Geometry check sheet. Reference: the model listing, model coordinates, mm. A direction names the side the tool comes from. Round coordinates to 2 decimals unless told otherwise and drop trailing zeros. Loops run counter-clockwise (first coordinate to the right, second up) from the corner with the lowest first, then second, coordinate; pieces in that order, holes last.
```python
from build123d import *

# Parameters (mm, degrees)
SKETCH1_W               = 68.58
SKETCH1_H               = 57.15
BOSS_EXTRUDE1_DEPTH     = 31.75
SKETCH2_W               = 26.162
SKETCH2_H               = 26.162
SKETCH2_W_2             = 26.67
SKETCH2_H_2             = 27.94
CUT_EXTRUDE1_DEPTH      = 95.749149864
SKETCH5_R               = 3.556
SKETCH5_R_2             = 3.729278609
CUT_EXTRUDE2_DEPTH      = 95.749149864
CUT_EXTRUDE3_START      = -16.51
CUT_EXTRUDE3_DEPTH      = 6.35
SKETCH7_R               = 5.334
CUT_EXTRUDE4_DEPTH      = 5.842
CUT_EXTRUDE5_DEPTH      = 7.62
SKETCH10_W              = 36.322
SKETCH10_H              = 6.35
CUT_EXTRUDE6_DEPTH      = 95.749149864
CUT_EXTRUDE7_DEPTH      = 87.293112332
CUT_EXTRUDE7_DEPTH_BACK = 87.293112332
SKETCH12_R              = 3.556
SKETCH13_R              = 5.334
CUT_EXTRUDE8_DEPTH      = 6.35
CUT_EXTRUDE9_DEPTH      = 7.62
CHAMFER1_SIZE           = 0.762
CHAMFER3_SIZE           = 3.81
CHAMFER5_SIZE           = 1.27
CHAMFER6_SIZE           = 2.54
CHAMFER9_SIZE           = 3.81
CHAMFER10_SIZE          = 6.35


# Some blends are built 0.0001 mm under size
with BuildPart() as part:
    # Sketch1 → Boss-Extrude1 (new body)
    with BuildSketch(Plane.XY):
        with Locations((34.29, 28.575)):
            Rectangle(SKETCH1_W, SKETCH1_H)
    extrude(amount=BOSS_EXTRUDE1_DEPTH)

    # Sketch2 → Cut-Extrude1 (cut, through all)
    with BuildSketch(Plane.XY.offset(31.75)):
        with Locations((19.431, 28.575)):
            Rectangle(SKETCH2_W, SKETCH2_H)
        with Locations((49.022, 28.575)):
            Rectangle(SKETCH2_W_2, SKETCH2_H_2)
    extrude(amount=-CUT_EXTRUDE1_DEPTH, mode=Mode.SUBTRACT)

    # Sketch5 → Cut-Extrude2 (cut, through all)
    with BuildSketch(Plane(origin=(68.58, 0, 0), x_dir=(0, 0, -1), z_dir=(1, 0, 0))):
        with Locations((-12.7, 47.625)):
            Circle(SKETCH5_R)
        with Locations((-12.7, 9.525)):
            Circle(SKETCH5_R_2)
    extrude(amount=-CUT_EXTRUDE2_DEPTH, mode=Mode.SUBTRACT)

    # Sketch6 → Cut-Extrude3 (cut)
    with BuildSketch(Plane(origin=(68.58, 0, 0), x_dir=(0, 0, -1), z_dir=(1, 0, 0)).offset(CUT_EXTRUDE3_START)):
        with BuildLine():
            Line((-21.59, 47.625), (-21.59, 12.21272508))
            ThreePointArc((-21.59, 12.21272508), (-15.38772508, 0.635), (-3.81, 6.83727492))
            Line((-3.81, 6.83727492), (-3.81, 47.625))
            ThreePointArc((-3.81, 47.625), (-12.7, 56.515), (-21.59, 47.625))
        make_face()
    extrude(amount=-CUT_EXTRUDE3_DEPTH, mode=Mode.SUBTRACT)

    # Sketch7 → Cut-Extrude4 (cut)
    with BuildSketch(Plane(origin=(68.58, 0, 0), x_dir=(0, 0, -1), z_dir=(1, 0, 0))):
        with Locations((-12.7, 47.625)):
            Circle(SKETCH7_R)
        with Locations((-12.7, 9.525)):
            Circle(SKETCH7_R)
    extrude(amount=-CUT_EXTRUDE4_DEPTH, mode=Mode.SUBTRACT)

    # Sketch9 → Cut-Extrude5 (cut)
    with BuildSketch(Plane.ZY):
        Polygon((16.072880273, 53.467), (9.327119727, 53.467), (5.954239455, 47.625), (9.327119727, 41.783), (16.072880273, 41.783), (19.445760545, 47.625), align=None)
        Polygon((16.072880273, 15.367), (9.327119727, 15.367), (5.954239455, 9.525), (9.327119727, 3.683), (16.072880273, 3.683), (19.445760545, 9.525), align=None)
    extrude(amount=-CUT_EXTRUDE5_DEPTH, mode=Mode.SUBTRACT)

    # Sketch10 → Cut-Extrude6 (cut, through all)
    with BuildSketch(Plane(origin=(0, 57.15, 0), x_dir=(1, 0, 0), z_dir=(0, 1, 0))):
        with Locations((50.419, -28.575)):
            Rectangle(SKETCH10_W, SKETCH10_H)
    extrude(amount=-CUT_EXTRUDE6_DEPTH, mode=Mode.SUBTRACT)

    # Sketch12 → Cut-Extrude7 (cut, two sides: drawn at the far end of the back side and taken through both)
    with BuildSketch(Plane(origin=(0, 15.494, 0), x_dir=(1, 0, 0), z_dir=(0, 1, 0)).offset(-CUT_EXTRUDE7_DEPTH_BACK)):
        with Locations(Location((19.431, -22.86, 0), (0, 0, 180))):
            Circle(SKETCH12_R)
    extrude(amount=CUT_EXTRUDE7_DEPTH + CUT_EXTRUDE7_DEPTH_BACK, mode=Mode.SUBTRACT)

    # Sketch13 → Cut-Extrude8 (cut)
    with BuildSketch(Plane(origin=(0, 57.15, 0), x_dir=(1, 0, 0), z_dir=(0, 1, 0))):
        with Locations(Location((19.431, -22.86, 0), (0, 0, 270))):
            Circle(SKETCH13_R)
    extrude(amount=-CUT_EXTRUDE8_DEPTH, mode=Mode.SUBTRACT)

    # Sketch14 → Cut-Extrude9 (cut)
    with BuildSketch(Plane.XZ):
        Polygon((22.803880273, 28.702), (16.058119727, 28.702), (12.685239455, 22.86), (16.058119727, 17.018), (22.803880273, 17.018), (26.176760545, 22.86), align=None)
    extrude(amount=-CUT_EXTRUDE9_DEPTH, mode=Mode.SUBTRACT)

    # Chamfer1
    chamfer1_edges = [part.edges().sort_by_distance(p)[0] for p in [
        (0, 50.546, 17.759320409),
        (0, 53.467, 12.7),
        (0, 50.546, 7.640679591),
        (0, 44.704, 7.640679591),
        (0, 41.783, 12.7),
        (0, 44.704, 17.759320409),
        (0, 12.446, 17.759320409),
        (0, 15.367, 12.7),
        (0, 12.446, 7.640679591),
        (0, 6.604, 7.640679591),
        (0, 3.683, 12.7),
        (0, 6.604, 17.759320409),
        (22.987, 41.656, 22.86),
        (22.987, 15.494, 22.86),
        (19.431, 57.15, 17.526),
        (24.490320409, 0, 25.781),
        (19.431, 0, 28.702),
        (14.371679591, 0, 25.781),
        (14.371679591, 0, 19.939),
        (19.431, 0, 17.018),
        (24.490320409, 0, 19.939),
        (45.72, 47.625, 16.256),
        (45.72, 9.525, 16.429278609),
        (52.07, 9.525, 16.429278609),
        (52.07, 47.625, 16.256),
        (68.58, 47.625, 18.034),
        (68.58, 9.525, 18.034),
    ]]
    chamfer(chamfer1_edges, length=CHAMFER1_SIZE)

    # Chamfer3
    chamfer3_edges = [part.edges().sort_by_distance(p)[0] for p in [
        (49.022, 42.545, 25.4),
        (49.022, 14.605, 25.4),
        (49.022, 42.545, 0),
        (49.022, 14.605, 0),
    ]]
    chamfer(chamfer3_edges, length=CHAMFER3_SIZE - 0.0001)  # a hair under: the kernel refuses the full size

    # Chamfer5
    chamfer5_edges = [part.edges().sort_by_distance(p)[0] for p in [
        (19.304, 41.656, 31.75),
        (32.258, 49.403, 31.75),
        (32.258, 7.747, 31.75),
        (35.687, 28.575, 25.4),
        (62.357, 28.575, 25.4),
        (6.35, 28.575, 0),
        (19.431, 41.656, 0),
        (32.512, 28.575, 0),
        (19.431, 15.494, 0),
        (6.35, 28.575, 31.75),
        (19.304, 15.494, 31.75),
        (35.687, 28.575, 0),
        (62.357, 28.575, 0),
    ]]
    chamfer(chamfer5_edges, length=CHAMFER5_SIZE)

    # Chamfer6
    chamfer6_edges = [part.edges().sort_by_distance(p)[0] for p in [
        (68.58, 57.15, 12.7),
        (68.58, 0, 12.7),
        (68.58, 28.575, 25.4),
        (0, 28.575, 31.75),
        (68.58, 28.575, 0),
        (0, 28.575, 0),
        (0, 57.15, 15.875),
        (0, 0, 15.875),
    ]]
    chamfer(chamfer6_edges, length=CHAMFER6_SIZE)

    # Chamfer9
    # the kernel refuses this chamfer: 3.81 mm, written as the material it takes off along each edge
    with BuildSketch(Plane(origin=(32.258, 57.15, 25.4), x_dir=(0, 0.027495876610586386, -0.9996219169112968), z_dir=(1, 0, 0))) as chamfer9_piece_1:
        Polygon((CHAMFER9_SIZE * 0.999621916911, -CHAMFER9_SIZE * 0.0274958766106), (-CHAMFER9_SIZE * 0.0274958766106, -CHAMFER9_SIZE * 0.999621916911), (0, 0), align=None)
    extrude(amount=43.580112184, mode=Mode.SUBTRACT)
    with BuildSketch(Plane(origin=(32.258, 57.15, 40.278112184), x_dir=(-0.9996219169112968, 0.027495876610586414, 0), z_dir=(0, 0, -1))) as chamfer9_piece_2:
        Polygon((CHAMFER9_SIZE * 0.999621916911, -CHAMFER9_SIZE * 0.0274958766106), (-CHAMFER9_SIZE * 0.0274958766106, -CHAMFER9_SIZE * 0.999621916911), (0, 0), align=None)
    extrude(amount=14.878112184, mode=Mode.SUBTRACT)
    with BuildSketch(Plane(origin=(40.786112184, 57.15, 31.75), x_dir=(0, 0.027495876610586386, -0.9996219169112968), z_dir=(-1, 0, 0)), Plane(origin=(-7.258112184, 0, 31.75), x_dir=(0, -0.027495876610586376, -0.9996219169112968), z_dir=(1, 0, 0))) as chamfer9_piece_3:
        Polygon((CHAMFER9_SIZE * 0.999621916911, CHAMFER9_SIZE * 0.0274958766106), (-CHAMFER9_SIZE * 0.0274958766106, CHAMFER9_SIZE * 0.999621916911), (0, 0), align=None)
    extrude(amount=48.044224368, mode=Mode.SUBTRACT)
    with BuildSketch(Plane(origin=(32.258, 0, 40.278112184), x_dir=(-0.9996219169112968, -0.02749587661058639, 0), z_dir=(0, 0, -1))) as chamfer9_piece_4:
        Polygon((CHAMFER9_SIZE * 0.999621916911, CHAMFER9_SIZE * 0.0274958766106), (-CHAMFER9_SIZE * 0.0274958766106, CHAMFER9_SIZE * 0.999621916911), (0, 0), align=None)
    extrude(amount=14.878112184, mode=Mode.SUBTRACT)
    with BuildSketch(Plane(origin=(32.258, 0, 25.4), x_dir=(0, -0.027495876610586403, -0.9996219169112968), z_dir=(1, 0, 0))) as chamfer9_piece_5:
        Polygon((CHAMFER9_SIZE * 0.999621916911, CHAMFER9_SIZE * 0.0274958766106), (-CHAMFER9_SIZE * 0.0274958766106, CHAMFER9_SIZE * 0.999621916911), (0, 0), align=None)
    extrude(amount=43.580112184, mode=Mode.SUBTRACT)
    with BuildSketch(Plane(origin=(32.258, 57.15, 40.278112184), x_dir=(-0.9996219169112968, 0.027495876610586414, 0), z_dir=(0, 0, -1))) as chamfer9_piece_6a_section:
        Polygon((CHAMFER9_SIZE * 0.999621916911, -CHAMFER9_SIZE * 0.0274958766106), (-CHAMFER9_SIZE * 0.0274958766106, -CHAMFER9_SIZE * 0.999621916911), (0, 0), align=None)
    chamfer9_piece_6a = extrude(amount=24.676224368, mode=Mode.PRIVATE)
    chamfer9_piece_6a = split(chamfer9_piece_6a, bisect_by=Plane(origin=(31.001486282, 55.893486282, 25.4), z_dir=(0, 0, -1)), keep=Keep.TOP, mode=Mode.PRIVATE)
    with BuildSketch(Plane(origin=(22.459887816, 57.15, 25.4), x_dir=(0, 0.027495876610586386, -0.9996219169112968), z_dir=(1, 0, 0))) as chamfer9_piece_6b_section:
        Polygon((CHAMFER9_SIZE * 0.999621916911, -CHAMFER9_SIZE * 0.0274958766106), (-CHAMFER9_SIZE * 0.0274958766106, -CHAMFER9_SIZE * 0.999621916911), (0, 0), align=None)
    chamfer9_piece_6b = extrude(amount=53.378224368, mode=Mode.PRIVATE)
    chamfer9_piece_6b = split(chamfer9_piece_6b, bisect_by=Plane(origin=(32.258, 55.893486282, 24.143486282), z_dir=(-1, 0, 0)), keep=Keep.TOP, mode=Mode.PRIVATE)
    chamfer9_piece_6 = chamfer9_piece_6a & chamfer9_piece_6b
    add(chamfer9_piece_6, mode=Mode.SUBTRACT)
    with BuildSketch(Plane(origin=(32.258, 0, 40.278112184), x_dir=(-0.9996219169112968, -0.02749587661058639, 0), z_dir=(0, 0, -1))) as chamfer9_piece_7a_section:
        Polygon((CHAMFER9_SIZE * 0.999621916911, CHAMFER9_SIZE * 0.0274958766106), (-CHAMFER9_SIZE * 0.0274958766106, CHAMFER9_SIZE * 0.999621916911), (0, 0), align=None)
    chamfer9_piece_7a = extrude(amount=24.676224368, mode=Mode.PRIVATE)
    chamfer9_piece_7a = split(chamfer9_piece_7a, bisect_by=Plane(origin=(31.001486282, 1.256513718, 25.4), z_dir=(0, 0, -1)), keep=Keep.TOP, mode=Mode.PRIVATE)
    with BuildSketch(Plane(origin=(22.459887816, 0, 25.4), x_dir=(0, -0.02749587661058639, -0.9996219169112968), z_dir=(1, 0, 0))) as chamfer9_piece_7b_section:
        Polygon((CHAMFER9_SIZE * 0.999621916911, CHAMFER9_SIZE * 0.0274958766106), (-CHAMFER9_SIZE * 0.0274958766106, CHAMFER9_SIZE * 0.999621916911), (0, 0), align=None)
    chamfer9_piece_7b = extrude(amount=53.378224368, mode=Mode.PRIVATE)
    chamfer9_piece_7b = split(chamfer9_piece_7b, bisect_by=Plane(origin=(32.258, 1.256513718, 24.143486282), z_dir=(-1, 0, 0)), keep=Keep.TOP, mode=Mode.PRIVATE)
    chamfer9_piece_7 = chamfer9_piece_7a & chamfer9_piece_7b
    add(chamfer9_piece_7, mode=Mode.SUBTRACT)

    # Chamfer10
    # the kernel refuses this chamfer: 6.35 mm, written as the material it takes off along each edge
    with BuildSketch(Plane(origin=(82.370186974, 57.15, 0), x_dir=(0, -0.9996219169112968, -0.027495876610586355), z_dir=(-1, 0, 0)), Plane(origin=(-13.790186974, 0, 0), x_dir=(0, 0.9996219169112966, -0.02749587661058638), z_dir=(1, 0, 0))) as chamfer10_piece_1:
        Polygon((CHAMFER10_SIZE * 0.999621916911, CHAMFER10_SIZE * 0.0274958766106), (-CHAMFER10_SIZE * 0.0274958766106, CHAMFER10_SIZE * 0.999621916911), (0, 0), align=None)
    extrude(amount=96.160373947, mode=Mode.SUBTRACT)


solid = part.part
```
1) Access from +Z, -Z, +X, -X, +Y, -Y to the whole of each face (thin tool, end or side, straight path). Record for faces 1 (the face through (49, 11, 3.81)), 2 (the face through (32.512, 28, 14)), 3 (the face through (0.386, 50.688, 18.111)), 4 (the face through (19, 4, 17.018)), 5 (the face through (62.738, 47, 9)).
Report:
face 1: none
face 2: +Z, -Z
face 3: -X
face 4: -Y
face 5: +X
2) Scan lines: line 1 along Y through (x, z) = (62.5, 12.5); line 2 along X through (y, z) = (19.5, 22); line 3 along Y through (x, z) = (38.5, 13) (3 decimals). Record each from-to range of solid material in increasing order.
Report:
line 1: y = 0 to 5.8, 13.25 to 44.07, 51.18 to 57.15
line 2: x = 0 to 6.35, 32.51 to 35.69, 62.36 to 68.58
line 3: y = 0 to 5.808, 13.242 to 14.605, 42.545 to 44.082, 51.168 to 57.15
3) Mould release check, pull along Y, two halves, no side actions. Record for faces 6 (the face through (4.143, 50.587, 7.664)), 7 (the face through (34.8, 53.9, 3.1)), 8 (the face through (33.81, 3.22, 3.13)): +Y half, -Y half, draft (parallel to the pull), parting line (faces both ways), or undercut.
Report:
face 6: undercut
face 7: +Y half
face 8: -Y half
4) Sectioned sample at D-D, the plane x = 30. Record the cut outline in (y, z) (3 decimals).
Report:
outline: (0, 6.35) - (6.35, 0) - (14.224, 0) - (15.494, 1.27) - (15.494, 30.48) - (14.224, 31.75) - (3.81, 31.75) - (1.552, 29.492) - (1.552, 23.142) - (0, 21.59) - close; (41.656, 1.27) - (42.926, 0) - (50.8, 0) - (57.15, 6.35) - (57.15, 21.59) - (55.598, 23.142) - (55.598, 29.492) - (53.34, 31.75) - (42.926, 31.75) - (41.656, 30.48) - close; hole circle Ø7.459 at (9.525, 12.7); hole circle Ø7.112 at (47.625, 12.7)
5) Sectioned sample at B-B, the plane y = 26. Record the cut outline in (x, z).
Report:
outline: (0, 2.54) - (2.54, 0) - (5.08, 0) - (6.35, 1.27) - (6.35, 30.48) - (5.08, 31.75) - (2.54, 31.75) - (0, 29.21) - close; (32.51, 1.27) - (33.78, 0) - (34.42, 0) - (35.69, 1.27) - (35.69, 24.13) - (34.42, 25.4) - (32.51, 25.4) - close; (62.36, 1.27) - (63.63, 0) - (66.04, 0) - (68.58, 2.54) - (68.58, 22.86) - (66.04, 25.4) - (63.63, 25.4) - (62.36, 24.13) - close
6) Sectioned sample at C-C, the plane z = 12.7. State how many separate pieces and enclosed holes the cut face has, then the cut area to 3 significant figures.
Report:
separate pieces: 4
enclosed holes: 1
area: 1,280 mm2
7) Gauge pin test, flat ends, axial feed: pin 1 (6 mm diameter, centred on y = 9.525, z = 12.7, fed in from -X); pin 2 (5 mm diameter, centred on x = 50, y = 9, fed in from +Z); pin 3 (4 mm diameter, centred on y = 46.5, z = 28, fed in from +X); pin 4 (2 mm diameter, centred on x = 20, y = 2.5, fed in from -Z). Record the tip position at first contact, or that the pin passes through.
Report:
pin 1: passes through
pin 2: stops at z = 25.4
pin 3: stops at x = 32.26
pin 4: stops at z = 2.85
8) Sectioned sample at A-A, the plane x = 57. Record the cut outline in (y, z) (3 decimals), then the cut area to 3 significant figures.
Report:
outline: (0, 6.35) - (6.35, 0) - (10.795, 0) - (14.605, 3.81) - (14.605, 21.59) - (10.795, 25.4) - (3.81, 25.4) - (0, 21.59) - close; (42.545, 3.81) - (46.355, 0) - (50.8, 0) - (57.15, 6.35) - (57.15, 21.59) - (53.34, 25.4) - (46.355, 25.4) - (42.545, 21.59) - close; hole circle Ø7.459 at (9.525, 12.7); hole circle Ø7.112 at (47.625, 12.7)
area: 575 mm2
